Part model, mm, in its own coordinate system. Face numbers are marked on the shaded views. Round coordinates to 2 decimals unless told otherwise and drop trailing zeros. Write each loop counter-clockwise with the first axis right and the second up, starting at its lowest first coordinate (ties: lowest second). Pieces come first, ordered by that corner, then holes.
1) Pull direction Z, two halves, no side cores. Call the marked faces 1, 2, 3 and 4: +Z half, -Z half, draft (parallel to the pull), parting line (faces both ways), or undercut.
2) Flat gauge pins, fed straight in: pin 1 (2.5 mm diameter, centred on y = 0, z = -38.1, fed in from -X); pin 2 (4 mm diameter, centred on y = -2.5, z = 5.5, fed in from +X); pin 3 (2.5 mm diameter, centred on y = 0, z = 38.1, fed in from +X). Where does each tip first touch, or does it go through?
3) Drill centre lines: L1, parallel to Z at x = -33, y = -1; L2, parallel to X at y = -2.25, z = 0; L3, parallel to Z at x = -1, y = 1.25. Where is each one in solid material? Low to high.
4) Saw through at C-C on z = 29.5. Write the cut outline in (x, y), and give its area (3 significant figures).
5) Saw through at A-A on x = -28. Write the cut outline in (y, z), and give its area (3 significant figures).
6) Saw through at B-B on x = 20. Write the cut outline in (y, z).
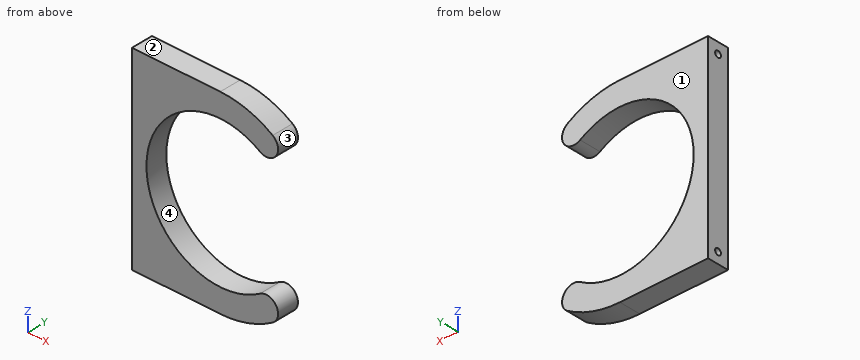
```python
from build123d import *

# Parameters (mm, degrees)
BOSS_EXTRUDE1_DEPTH = 4.7625
SKETCH2_R           = 1.3890625
CUT_EXTRUDE1_DEPTH  = 25.4


with BuildPart() as part:
    # Sketch1 → Boss-Extrude1 (new body, symmetric)
    with BuildSketch(Plane(origin=(0, 0, 0), x_dir=(1, 0, 0), z_dir=(0, 1, 0))):
        with BuildLine():
            Line((-38.862, 42.8625), (-38.862, -42.8625))
            Line((-38.862, -42.8625), (0, -42.8625))
            ThreePointArc((0, -42.8625), (12.029787175, -41.139739022), (23.092554324, -36.109941028))
            ThreePointArc((23.092554324, -36.109941028), (24.664283237, -28.961787885), (17.516130095, -27.390058972))
            ThreePointArc((17.516130095, -27.390058972), (-32.512, 0), (17.516130095, 27.390058972))
            ThreePointArc((17.516130095, 27.390058972), (24.664283237, 28.961787885), (23.092554324, 36.109941028))
            ThreePointArc((23.092554324, 36.109941028), (12.029787175, 41.139739022), (0, 42.8625))
            Line((0, 42.8625), (-38.862, 42.8625))
        make_face()
    extrude(amount=BOSS_EXTRUDE1_DEPTH, both=True)

    # Sketch2 → Cut-Extrude1 (cut)
    with BuildSketch(Plane.ZY.offset(38.862)):
        with Locations((-38.1, 0)):
            Circle(SKETCH2_R)
        with Locations((38.1, 0)):
            Circle(SKETCH2_R)
    extrude(amount=-CUT_EXTRUDE1_DEPTH, mode=Mode.SUBTRACT)


solid = part.part
```
Completed:
1. face 1: draft
1. face 2: +Z half
1. face 3: undercut
1. face 4: undercut
2. pin 1: stops at x = -13.46
2. pin 2: stops at x = -31.64
2. pin 3: stops at x = 21.89
3. L1: z = -42.86 to -39.06, -37.14 to 37.14, 39.06 to 42.86
3. L2: x = -38.86 to -32.51
3. L3: z = -42.86 to -32.5, 32.5 to 42.86
4. outline: (-38.86, -4.76) - (-13.67, -4.76) - (-13.67, 4.76) - (-38.86, 4.76) - close; (13.67, -4.76) - (24.96, -4.76) - (24.96, 4.76) - (13.67, 4.76) - close
4. area: 348 mm2
5. outline: (-4.76, -42.86) - (4.76, -42.86) - (4.76, -16.52) - (-4.76, -16.52) - close; (-4.76, 16.52) - (4.76, 16.52) - (4.76, 42.86) - (-4.76, 42.86) - close; hole circle Ø2.78 at (0, -38.1); hole circle Ø2.78 at (0, 38.1)
5. area: 490 mm2
6. outline: (-4.76, -37.91) - (4.76, -37.91) - (4.76, -26.58) - (-4.76, -26.58) - close; (-4.76, 26.58) - (4.76, 26.58) - (4.76, 37.91) - (-4.76, 37.91) - close
